Design review of the part shown in the three views and the two pictorial views. Dimensions are in mm from the part's minimum x, y and z. A direction names the side the tool comes from. Give positions to 0.01 mm unless a question says otherwise; leave off trailing zeros. Loops run counter-clockwise (first coordinate to the right, second up) from the corner with the lowest first, then second, coordinate; pieces in that order, holes last. Notation, with made-up numbers: (-0.75, 6) -> (47.25, 6) arc R30 cw to (47.25, 30) -> close; hole circle Ø10 at (88.5, 26.25). An arc over 180 degrees is marked (long way). One line per question, with ' | ' between items. Start each with the question number.
(1) Consider section B-B (x = 219.5). Write out the cut boundary in (y, z).
(2) Consider section A-A (y = 1624). Write out the cut boundary in (x, z), and give its area (3 significant figures).
(3) Insertion check: P1, Ø25, axis at x = 239.5, z = 97.5, coming from the +Y side; P2, Ø4, axis at y = 401.5, z = 106.5, coming from the -X side; P3, Ø4, axis at x = 232.5, y = 383.5, coming from the -Z side. Each pin has a flat end and moves straight along its axis. Give the tip position at first contact, or say it passes through.
(4) Tool access review of the marked faces 3, 4, 5 and 6: name each direction out of +Z, -Z, +X, -X, +Y, -Y from which nothing blocks a thin tool from reaching the whole face with its end or side.
(5) Draft analysis for pull direction X (two halves, no side actions). For the marked faces 1 and 2, state which applies: +X half, -X half, draft (parallel to the pull), parting line (faces both ways), or undercut.
(6) Consider section C-C (x = 50). Write out the cut boundary in (y, z).
(7) Wall thickness on probe 1 along Y at (x, z) = (324.5, 116); probe 2 along Z at (x, y) = (106, 1402.5); probe 3 along Z at (x, y) = (209.5, 1116): over which ranges is each line inside the solid? List them lowest first.
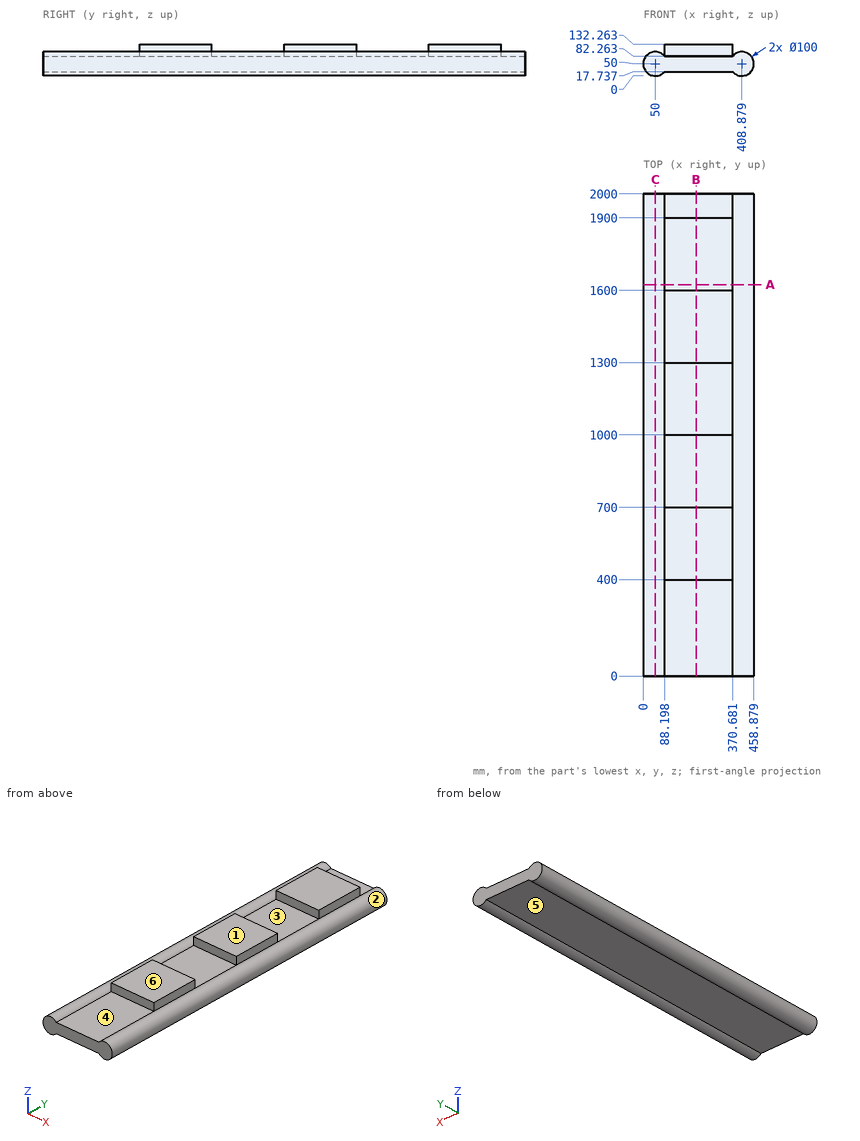
A:
1) outline: (0, 17.74) -> (2000, 17.74) -> (2000, 82.26) -> (1900, 82.26) -> (1900, 132.26) -> (1600, 132.26) -> (1600, 82.26) -> (1300, 82.26) -> (1300, 132.26) -> (1000, 132.26) -> (1000, 82.26) -> (700, 82.26) -> (700, 132.26) -> (400, 132.26) -> (400, 82.26) -> (0, 82.26) -> close
2) outline: (88.2, 17.74) -> (370.68, 17.74) arc R50 ccw (long way) to (370.68, 82.26) -> (370.68, 132.26) -> (88.2, 132.26) -> (88.2, 82.26) arc R50 ccw (long way) to start | area: 47,000 mm^2
3) P1: stops at y = 1900 | P2: stops at x = 88.2 | P3: stops at z = 17.74
4) face 3: +Z | face 4: +Z, -Y | face 5: -Z, +Y, -Y | face 6: +Z, +X, -X, +Y, -Y
5) face 1: draft | face 2: undercut
6) outline: (0, 0) -> (2000, 0) -> (2000, 100) -> (0, 100) -> close
7) probe 1: y = 400 to 700, 1000 to 1300, 1600 to 1900 | probe 2: z = 17.74 to 82.26 | probe 3: z = 17.74 to 132.26
